The listing builds one solid part. Answer for the finished solid, in the listing's coordinates (mm). Face numbers are marked on the shaded views. A direction names the side the tool comes from. Coordinates: 2 decimals unless noted, no trailing zeros. Loops run counter-clockwise (first coordinate to the right, second up) from the corner with the lowest first, then second, coordinate; pieces in that order, holes last. Notation, with made-up numbers: (-27, 65) - (16, 65) arc R14 ccw to (16, 73) - close; hole circle Ø3 at (28.5, 34). An arc over 180 degrees is marked (long way). One line per question, with ' | ' between items.
from build123d import *

# Parameters (mm, degrees)
F3_DEPTH = 6
F4_R     = 5
F5_DEPTH = 16
F6_R     = 2.5
F7_DEPTH = 25


with BuildPart() as f1:
    # F0 (on Front) → F1 (revolve)
    with BuildSketch(Plane.XZ):
        with BuildLine():
            ThreePointArc((0, 0), (10, 10), (0, 20))
            Line((0, 20), (0, 0))
        make_face()
    revolve(axis=Axis((0, 0, 10), (0, 0, -1)))

    # F2 (on Top) → F3 (cut)
    with BuildSketch(Plane.XY):
        Polygon((-2.598076, -4.5), (2.598076, -4.5), (5.196152, 0), (2.598076, 4.5), (-2.598076, 4.5), (-5.196152, 0), align=None)
    extrude(amount=F3_DEPTH, mode=Mode.SUBTRACT)

    # F4 (on face) → F5 (join)
    with BuildSketch(Plane(origin=(0, 0, 6), x_dir=(1, 0, 0), z_dir=(0, 0, -1))):
        Circle(F4_R)
    extrude(amount=-F5_DEPTH)

    # F6 (on face) → F7 (cut)
    with BuildSketch(Plane(origin=(0, 0, 6), x_dir=(1, 0, 0), z_dir=(0, 0, -1))):
        Circle(F6_R)
    extrude(amount=-F7_DEPTH, mode=Mode.SUBTRACT)


solid = f1.part
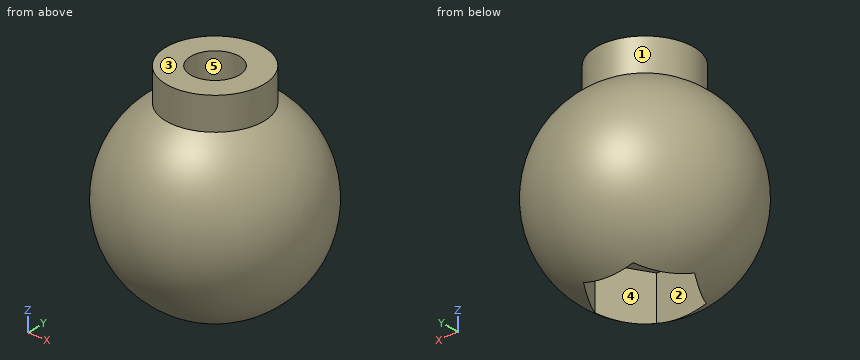
Item 1: Find section A-A, the plane x = 0. Write down the section's boundary in (y, z).
Taken from the geometry:
outline: (-5, 18.66) arc R10 ccw to (-4.5, 1.07) - (-4.5, 6) - (-2.5, 6) - (-2.5, 22) - (-5, 22) - close; (2.5, 6) - (4.5, 6) - (4.5, 1.07) arc R10 ccw to (5, 18.66) - (5, 22) - (2.5, 22) - close
Item 2: Which of the six approach directions +Z, -Z, +X, -X, +Y, -Y give full straight-line access (tool end or side, diameter ignored) to the marked faces 4 and 5?
Taken from the geometry:
face 4: -Z | face 5: +Z, -Z
Item 3: Find the intervals of material crossed by line 1 (Y direction, x = -2.25, z = 5); line 2 (X direction, y = -2.25, z = 14.5); line 3 (Z direction, x = 4.25, y = -0.5), in increasing order. Write a range as [from, to].
Taken from the geometry:
line 1: y = [-8.36, -4.5], [4.5, 8.36] | line 2: x = [-8.64, -1.09], [1.09, 8.64] | line 3: z = [6, 22]
Item 4: Each of these flat-tipped pins is pushed along its axis until it touches: pin 1 Ø8 at (y, z) = (6, 15) entering from -X; pin 2 Ø2 at (y, z) = (-2.5, 6.5) entering from -X; pin 3 Ø5 at (y, z) = (3.5, 13) entering from +X. Where does it stop, or does it pass through?
Taken from the geometry:
pin 1: stops at x = -9.25 | pin 2: stops at x = -9.44 | pin 3: stops at x = 9.77
Item 5: Find section D-D, the plane z = 20.5. Write down the section's boundary in (x, y).
Taken from the geometry:
outline: circle Ø10 at (0, 0); hole circle Ø5 at (0, 0)
Item 6: Find section B-B, the plane z = 4. Write down the section's boundary in (x, y).
Taken from the geometry:
outline: circle Ø16 at (0, 0); hole (-5.2, 0) - (-2.6, -4.5) - (2.6, -4.5) - (5.2, 0) - (2.6, 4.5) - (-2.6, 4.5) - close
Item 7: The mould has two halves that part along X. Classify the marked faces 1, 2 and 3: pulls with the +X half, pulls with the -X half, needs draft (parallel to the pull), parting line crosses it, or undercut.
Taken from the geometry:
face 1: parting line crosses it | face 2: undercut | face 3: needs draft
Item 8: Find section C-C, the plane y = -1.5. Write down the section's boundary in (x, z).
Taken from the geometry:
outline: (-4.77, 18.66) arc R9.89 ccw to (-4.33, 1.11) - (-4.33, 6) - (-2, 6) - (-2, 22) - (-4.77, 22) - close; (2, 6) - (4.33, 6) - (4.33, 1.11) arc R9.89 ccw to (4.77, 18.66) - (4.77, 22) - (2, 22) - close
